Geometry check sheet. Reference: drawing and pictorial views, mm from the part's lowest x, y, z. A direction names the side the tool comes from. Round coordinates to 2 decimals unless told otherwise and drop trailing zeros. Loops run counter-clockwise (first coordinate to the right, second up) from the corner with the lowest first, then second, coordinate; pieces in that order, holes last. Notation, with made-up numbers: (55, -5.75) -> (90, -5.75) arc R30 ccw to (90, 17.25) -> close; hole circle Ø2 at (25, -19). An arc over 180 degrees is marked (long way). Use one line per item in the form item = value. Start each with the question number.
(1) Material ranges on probe 1 along Y at (x, z) = (7.5, 1.95); probe 2 along Y at (x, z) = (2.5, 2.8); probe 3 along Y at (x, z) = (20, 2.3), recorded low to high. Write a range as [from, to].
(2) Sectioned sample at D-D (x = 7.5). Record the cut outline in (y, z).
(3) Sectioned sample at C-C (z = 1.3). Record the cut outline in (x, y), and give its area (3 significant figures).
(4) Set-up check for the marked faces 4 and 5: record each of +Z, -Z, +X, -X, +Y, -Y from which the full face is reachable in a straight line by a thin tool's end or side.
(5) Draft check along Y on the marked faces 1, 2 and 3. Enter one of: released by +Y, released by -Y, zero draft, split by the parting line, or undercut.
(6) Sectioned sample at A-A (y = 12.5). Record the cut outline in (x, z), and give its area (3 significant figures).
(7) Sectioned sample at B-B (x = 20). Record the cut outline in (y, z), and give its area (3 significant figures).
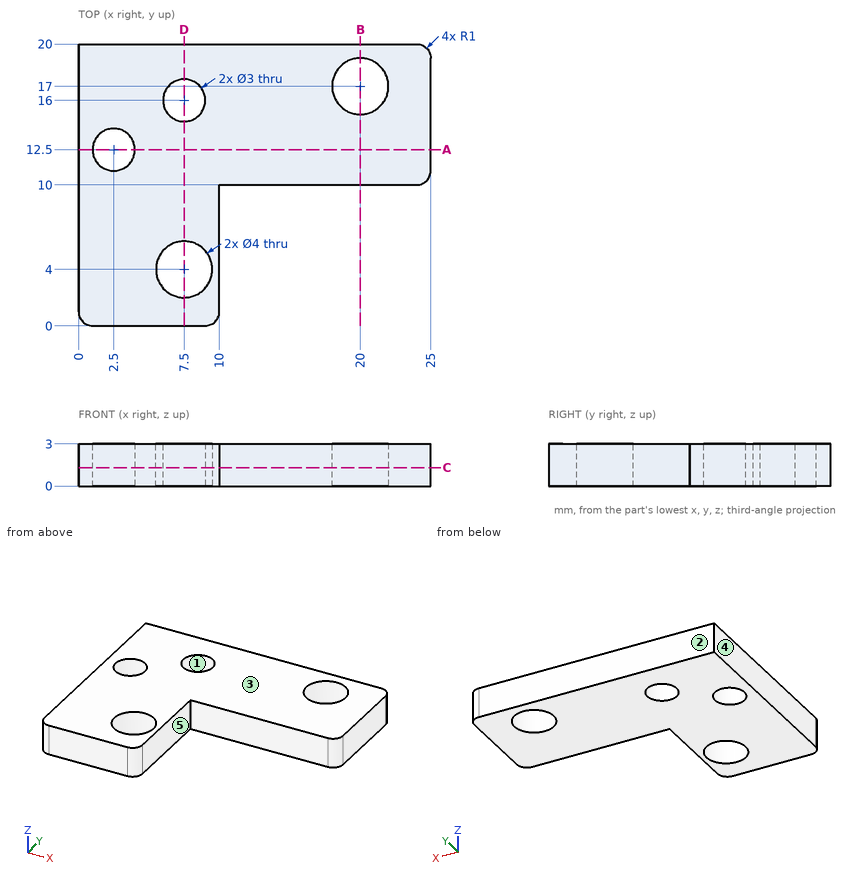
Checks:
q1.probe_1 = [0, 2], [6, 14.5], [17.5, 20]
q1.probe_2 = [0, 11], [14, 20]
q1.probe_3 = [10, 15], [19, 20]
q2.outline = (0, 0) -> (2, 0) -> (2, 3) -> (0, 3) -> close; (6, 0) -> (14.5, 0) -> (14.5, 3) -> (6, 3) -> close; (17.5, 0) -> (20, 0) -> (20, 3) -> (17.5, 3) -> close
q3.outline = (0, 1) arc R1 ccw to (1, 0) -> (9, 0) arc R1 ccw to (10, 1) -> (10, 10) -> (24, 10) arc R1 ccw to (25, 11) -> (25, 19) arc R1 ccw to (24, 20) -> (0, 20) -> close; hole circle Ø3 at (2.5, 12.5); hole circle Ø4 at (7.5, 4); hole circle Ø3 at (7.5, 16); hole circle Ø4 at (20, 17)
q3.area = 310 mm2
q4.face_4 = +Z, -Z, -X, +Y, -Y
q4.face_5 = +Z, -Z, +X, -Y
q5.face_1 = undercut
q5.face_2 = released by +Y
q5.face_3 = zero draft
q6.outline = (0, 0) -> (1, 0) -> (1, 3) -> (0, 3) -> close; (4, 0) -> (25, 0) -> (25, 3) -> (4, 3) -> close
q6.area = 66.0 mm2
q7.outline = (10, 0) -> (15, 0) -> (15, 3) -> (10, 3) -> close; (19, 0) -> (20, 0) -> (20, 3) -> (19, 3) -> close
q7.area = 18.0 mm2
